from build123d import *

# Parameters (mm, degrees)
BASE_SKETCH_W       = 3.2
BASE_SKETCH_H       = 10
BOSS_EXTRUDE1_DEPTH = 3.2
FILLET1_R           = 2


with BuildPart() as part:
    # Base_Sketch → Boss-Extrude1 (new body)
    with BuildSketch(Plane(origin=(0, 0, 0), x_dir=(1, 0, 0), z_dir=(0, 1, 0))):
        Polygon((-60, 15), (60, 15), (60, 5), (63.2, 5), (63.2, -5), (60, -5), (60, -15), (-60, -15), align=None)
        with Locations((-14.466666667, 0)):
            Rectangle(BASE_SKETCH_W, BASE_SKETCH_H, mode=Mode.SUBTRACT)
        with Locations((-43.4, 0)):
            Rectangle(BASE_SKETCH_W, BASE_SKETCH_H, mode=Mode.SUBTRACT)
        with Locations((14.466666667, 0)):
            Rectangle(BASE_SKETCH_W, BASE_SKETCH_H, mode=Mode.SUBTRACT)
        with Locations((43.4, 0)):
            Rectangle(BASE_SKETCH_W, BASE_SKETCH_H, mode=Mode.SUBTRACT)
    extrude(amount=BOSS_EXTRUDE1_DEPTH)

    # Fillet1
    fillet1_edges = [part.edges().sort_by_distance(p)[0] for p in [
        (-60, 1.6, 15),
        (-60, 1.6, -15),
    ]]
    fillet(fillet1_edges, radius=FILLET1_R)


solid = part.part
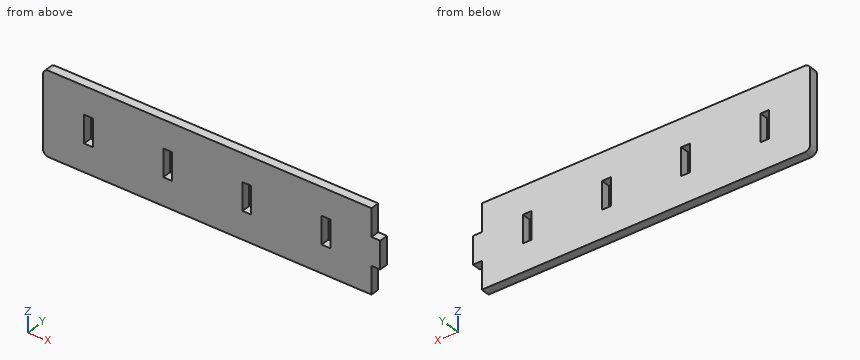
Can you work these out from the model? Positions are in its coordinate system, mm. Coordinates: 2 decimals unless noted, no trailing zeros. Loops run counter-clockwise (first coordinate to the right, second up) from the corner with the lowest first, then second, coordinate; pieces in that order, holes last. Notation, with made-up numbers: (77.25, -5) - (117.25, -5) arc R24 ccw to (117.25, 8) - close; hole circle Ø1 at (17.25, 87.25). An arc over 180 degrees is marked (long way). Answer as a JSON object with one key per item and string values. Group by question number.
Item 1: If we section it at B-B (z = -1): List the corners of the cut face in (x, y) for me.
Item 2: If I drill on L1, parallel to X at y = 1.35, z = 1; L2, parallel to Z at x = -42, y = 1.1; L3, parallel to X at y = 0.55, z = -10.5, over which ranges is the centre line in solid material (lowest first)? Write a range as from..to.
Item 3: For pin 1 (6 mm diameter, centred on x = 45, z = -10, fed in from -Y); pin 2 (1.5 mm diameter, centred on y = 2.5, z = -7, fed in from +X), each with a flat end and sliding along its axis, tell me the tip position at first contact or that it passes through.
Item 4: If we section it at D-D (z = 6.5): List the corners of the cut face in (x, y) for me, plus the area to 3 significant figures.
Item 5: If we section it at C-C (x = 14): List the corners of the cut face in (y, z) for me.
Item 6: If we section it at A-A (y = 1.1): List the corners of the cut face in (x, z) for me, plus the area to 3 significant figures.
Returned:
{
 "1": {"outline": "(-60, 0) - (-45, 0) - (-45, 3.2) - (-60, 3.2) - close; (-41.8, 0) - (-16.07, 0) - (-16.07, 3.2) - (-41.8, 3.2) - close; (-12.87, 0) - (12.87, 0) - (12.87, 3.2) - (-12.87, 3.2) - close; (16.07, 0) - (41.8, 0) - (41.8, 3.2) - (16.07, 3.2) - close; (45, 0) - (63.2, 0) - (63.2, 3.2) - (45, 3.2) - close"},
 "2": {"L1": "x = -60..-45, -41.8..-16.07, -12.87..12.87, 16.07..41.8, 45..63.2", "L2": "z = -15..-5, 5..15", "L3": "x = -60..60"},
 "3": {"pin 1": "stops at y = 0", "pin 2": "stops at x = 60"},
 "4": {"outline": "(-60, 0) - (60, 0) - (60, 3.2) - (-60, 3.2) - close", "area": "384 mm²"},
 "5": {"outline": "(0, -15) - (3.2, -15) - (3.2, -5) - (0, -5) - close; (0, 5) - (3.2, 5) - (3.2, 15) - (0, 15) - close"},
 "6": {"outline": "(-60, -13) arc R2 ccw to (-58, -15) - (60, -15) - (60, -5) - (63.2, -5) - (63.2, 5) - (60, 5) - (60, 15) - (-58, 15) arc R2 ccw to (-60, 13) - close; hole (-45, -5) - (-41.8, -5) - (-41.8, 5) - (-45, 5) - close; hole (-16.07, -5) - (-12.87, -5) - (-12.87, 5) - (-16.07, 5) - close; hole (12.87, -5) - (16.07, -5) - (16.07, 5) - (12.87, 5) - close; hole (41.8, -5) - (45, -5) - (45, 5) - (41.8, 5) - close", "area": "3,500 mm²"}
}
